Geometry check sheet. Reference: the model listing, model coordinates, mm. A direction names the side the tool comes from. Give positions to 0.01 mm unless a question says otherwise; leave off trailing zeros. Order: outer loops, then holes, each group sorted by start corner. A loop starts at its lowest first (then second) coordinate and runs counter-clockwise, first axis right, second up. Notation, with made-up numbers: M 83,61.5 L 138,61.5 A24 cw 138,77.5 Z; hole C -24.75,-28 d2. An arc over 180 degrees is marked long. Answer as CSV lines item,"result".
from build123d import *

# Parameters (mm, degrees)
SKETCH_1_R      = 1.5
EXTRUDE_1_DEPTH = 3
FILLET_1_R      = 1


with BuildPart() as part:
    # 草图1 → 凸台-拉伸1 (new body)
    with BuildSketch(Plane(origin=(0, 0, 0), x_dir=(1, 0, 0), z_dir=(0, 1, 0))):
        Polygon((0, 10.5), (0, -10.5), (5, -10.5), (5, -7.5), (15, -7.5), (15, -10.5), (35, -10.5), (35, -7.5), (45, -7.5), (45, -10.5), (50, -10.5), (50, 10.5), (45, 10.5), (45, 7.5), (35, 7.5), (35, 10.5), (15, 10.5), (15, 7.5), (5, 7.5), (5, 10.5), align=None)
        with Locations(Location((10, 0, 0), (0, 0, 270))):
            Circle(SKETCH_1_R, mode=Mode.SUBTRACT)
        with Locations(Location((40, 0, 0), (0, 0, 270))):
            Circle(SKETCH_1_R, mode=Mode.SUBTRACT)
        with Locations(Location((25, 0, 0), (0, 0, 270))):
            Circle(SKETCH_1_R, mode=Mode.SUBTRACT)
    extrude(amount=EXTRUDE_1_DEPTH)

    # 圆角1
    fillet_1_edges = [part.edges().sort_by_distance(p)[0] for p in [
        (0, 1.5, 10.5),
        (0, 1.5, -10.5),
        (5, 1.5, -10.5),
        (15, 1.5, -10.5),
        (35, 1.5, -10.5),
        (45, 1.5, -10.5),
        (50, 1.5, -10.5),
        (50, 1.5, 10.5),
        (45, 1.5, 10.5),
        (35, 1.5, 10.5),
        (15, 1.5, 10.5),
        (5, 1.5, 10.5),
    ]]
    fillet(fillet_1_edges, radius=FILLET_1_R)


solid = part.part
(1) Section check A-A on x = 25. Enter the section's corners in (y, z).
The answers:
outline,"M 0,-10.5 L 3,-10.5 L 3,-1.5 L 0,-1.5 Z; M 0,1.5 L 3,1.5 L 3,10.5 L 0,10.5 Z"
(2) Material ranges on line 1 (X direction, y = 1.75, z = 0); line 2 (Z direction, x = 14.5, y = 1.6); line 3 (Z direction, x = 10.5, y = 2.2), recorded low to high.
The answers:
line 1,"x = 0 to 8.5, 11.5 to 23.5, 26.5 to 38.5, 41.5 to 50"
line 2,"z = -7.5 to 7.5"
line 3,"z = -7.5 to -1.41, 1.41 to 7.5"
(3) Section check B-B on z = 8.5. Enter the section's corners in (x, y), then the cut area to 3 significant figures.
The answers:
outline,"M 0,0 L 5,0 L 5,3 L 0,3 Z; M 15,0 L 35,0 L 35,3 L 15,3 Z; M 45,0 L 50,0 L 50,3 L 45,3 Z"
area,"90.0 mm2"
(4) Tool access check on faces 1 (the face through (25, 0, -2)), 2 (the face through (4.699, 1.521, 10.215)), 3 (the face through (5, 1, -8)). Record the directions out of +Z, -Z, +X, -X, +Y, -Y that give a thin tool (end or side, any length) a straight path to the whole face; none if there is none.
The answers:
face 1,"+Z, -Z, +X, -X, -Y"
face 2,"+Z, +Y, -Y"
face 3,"-Z, +Y, -Y"
(5) Gauge pin test, flat ends, axial feed: P1, Ø1.8, axis at x = 40, z = 0, coming from the -Y side; P2, Ø1.5, axis at x = 40, y = 1.5, coming from the +Z side; P3, Ø0.9, axis at x = 41, y = 1, coming from the -Z side. Record the tip position at first contact, or that the pin passes through.
The answers:
P1,"passes through"
P2,"stops at z = 7.5"
P3,"stops at z = -7.5"
(6) Section check C-C on z = 0. Enter the section's corners in (x, y), then the cut area to 3 significant figures.
The answers:
outline,"M 0,0 L 8.5,0 L 8.5,3 L 0,3 Z; M 11.5,0 L 23.5,0 L 23.5,3 L 11.5,3 Z; M 26.5,0 L 38.5,0 L 38.5,3 L 26.5,3 Z; M 41.5,0 L 50,0 L 50,3 L 41.5,3 Z"
area,"123 mm2"
(7) Section check D-D on x = 10. Enter the section's corners in (y, z), then the cut area to 3 significant figures.
The answers:
outline,"M 0,-7.5 L 3,-7.5 L 3,-1.5 L 0,-1.5 Z; M 0,1.5 L 3,1.5 L 3,7.5 L 0,7.5 Z"
area,"36.0 mm2"
(8) Draft check along X on faces 4 (the face through (0.285, 1.521, -10.199)), 5 (the face through (45, 1, 8)), 6 (the face through (25, 3, -2)). Enter one of: +X half, -X half, draft (parallel to the pull), parting line (faces both ways), or undercut.
The answers:
face 4,"-X half"
face 5,"undercut"
face 6,"draft"
